```python
from build123d import *

# Parameters (mm, degrees)
BOSS_EXTRUDE1_DEPTH = 5
BOSS_EXTRUDE2_DEPTH = 5
SKETCH3_W           = 72.5
SKETCH3_H           = 27.5
CUT_EXTRUDE1_DEPTH  = 129.452325787
SKETCH4_R           = 1.5
CUT_EXTRUDE2_DEPTH  = 5
FILLET2_R           = 10
FILLET3_R           = 2
FILLET1_R           = 2


with BuildPart() as part:
    # Sketch1 → Boss-Extrude1 (new body)
    with BuildSketch(Plane(origin=(0, 0, 0), x_dir=(1, 0, 0), z_dir=(0, 1, 0))):
        with BuildLine():
            Line((0, -80), (100, -80))
            Line((100, -80), (100, -30))
            Line((100, -30), (74.161984871, -30))
            ThreePointArc((74.161984871, -30), (-44.72135955, 66.332495807), (0, -80))
        make_face()
    extrude(amount=BOSS_EXTRUDE1_DEPTH)

    # Sketch2 → Boss-Extrude2 (add)
    with BuildSketch(Plane.XZ):
        with BuildLine():
            Line((0, 74.8), (94.8, 74.8))
            Line((94.8, 74.8), (94.8, 35.2))
            Line((94.8, 35.2), (66, 35.2))
            ThreePointArc((66, 35.2), (-38.484282506, -64.140470843), (0, 74.8))
        make_face()
    extrude(amount=BOSS_EXTRUDE2_DEPTH)

    # Sketch3 → Cut-Extrude1 (cut, through all)
    with BuildSketch(Plane(origin=(0, 5, 0), x_dir=(1, 0, 0), z_dir=(0, 1, 0))):
        with Locations((0, 10)):
            Rectangle(SKETCH3_W, SKETCH3_H)
    extrude(amount=-CUT_EXTRUDE1_DEPTH, mode=Mode.SUBTRACT)

    # Sketch4 → Cut-Extrude2 (cut)
    with BuildSketch(Plane.XZ.offset(5)):
        with Locations(Location((-37.5, 5.5, 0), (0, 0, 270))):
            Circle(SKETCH4_R)
        with Locations(Location((37.5, 5.5, 0), (0, 0, 270))):
            Circle(SKETCH4_R)
        with Locations(Location((37.5, -25.5, 0), (0, 0, 270))):
            Circle(SKETCH4_R)
        with Locations(Location((-37.5, -25.5, 0), (0, 0, 270))):
            Circle(SKETCH4_R)
    extrude(amount=-CUT_EXTRUDE2_DEPTH, mode=Mode.SUBTRACT)

    # Fillet2
    fillet2_edges = [part.edges().sort_by_distance(p)[0] for p in [
        (66, -2.5, 35.2),
        (74.161984871, 2.5, 30),
    ]]
    fillet(fillet2_edges, radius=FILLET2_R)

    # Fillet3
    fillet3_edges = [part.edges().sort_by_distance(p)[0] for p in [
        (100, 5, 55),
        (93.874821937, 5, 30),
        (-49.888765157, 5, -62.538876798),
        (79.932284274, 5, 26.236095645),
        (50, 5, 80),
    ]]
    fillet(fillet3_edges, radius=FILLET3_R)

    # Fillet1
    fillet1_edges = [part.edges().sort_by_distance(p)[0] for p in [
        (-44.341645317, -5, -60.240007392),
        (94.8, -5, 55),
        (47.4, -5, 74.8),
        (87.88456496, -5, 35.2),
        (72.915652996, -5, 31.128027449),
    ]]
    fillet(fillet1_edges, radius=FILLET1_R)


solid = part.part
```
Read the model definition and answer for the solid it produces. Units are mm, in the model's axes. A direction names the side the tool comes from. Give positions to 0.01 mm unless a question says otherwise; leave off trailing zeros. Write item = value, one per line. Start each with the question number.
Item 1: Find the intervals of material crossed by probe 1 along X at (y, z) = (-1.7, -25.5); probe 2 along X at (y, z) = (-2, 5.5); probe 3 along Z at (x, y) = (8, 1.5), in increasing order. Write a range as [from, to].
Item 2: A tool of negligible diameter and unlimited length cuts with its end or side. For faces 1 (the cylindrical face through (72.99, -1.52, 31.23)), 2 (the flat face through (-1, 0, 3.75)), 3 (the flat face through (76, 0, 11)), from which of +Z, -Z, +X, -X, +Y, -Y can it reach the whole face along a straight path? Write none if from no direction.
Item 3: Each of these flat-tipped pins is pushed along its axis until it touches: P1, Ø2, axis at y = -3.5, z = -42.5, coming from the -X side; P2, Ø5, axis at y = 0.5, z = -38, coming from the +X side; P3, Ø3, axis at y = 0.5, z = -10, coming from the +X side. Where does it stop, or does it pass through?
Item 4: The mould has two halves that part along Z. Classify faces 4 (the flat face through (9, 5, 16)), 5 (the cylindrical face through (79.855, 1.521, 26.137)): +Z half, -Z half, draft (parallel to the pull), parting line (faces both ways), or undercut.
Response:
q1.probe_1 = [-70.32, -39], [-36, 36], [39, 70.32]
q1.probe_2 = [-74.6, -39], [-36, 36], [39, 74.6]
q1.probe_3 = [-79.6, -23.75], [3.75, 80]
q2.face_1 = +X, -Y
q2.face_2 = +Y, -Y
q2.face_3 = -Y
q3.P1 = -62.19
q3.P2 = 71.69
q3.P3 = 79.55
q4.face_4 = draft
q4.face_5 = undercut
